Here's how the part is built. I have some questions about the finished solid (model axes, mm). A direction names the side the tool comes from. Give positions to 0.01 mm unless a question says otherwise; leave off trailing zeros. Write each loop counter-clockwise with the first axis right and the second up, starting at its lowest first coordinate (ties: lowest second). Pieces come first, ordered by that corner, then holes. Notation, with made-up numbers: (27, -3) -> (46, -3) arc R25 ccw to (46, 18) -> close; hole circle Ø9 at (33.5, -4). An arc over 180 degrees is marked (long way). Use one line per item in the form item = value.
```python
from build123d import *

# Parameters (mm, degrees)
SKETCH_1_R           = 7.83
EXTRUDE_1_DEPTH      = 5.5
EXTRUDE_1_DEPTH_BACK = 5.5
SKETCH_3_R           = 9.5
EXTRUDE_3_DEPTH      = 1.5
SKETCH_4_R           = 9.5
EXTRUDE_4_DEPTH      = 1.5
SKETCH_5_R           = 3
CUT_EXTRUDE_1_DEPTH  = 15
SKETCH_6_R           = 2
CUT_EXTRUDE_2_DEPTH  = 10.5
SKETCH_7_R           = 2
CUT_EXTRUDE_3_DEPTH  = 10.5


with BuildPart() as part:
    # Sketch 1 → Extrude 1 (new body, two sides)
    with BuildSketch(Plane(origin=(0, 0, 0), x_dir=(1, 0, 0), z_dir=(0, 1, 0))) as extrude_1_sk:
        Circle(SKETCH_1_R)
    extrude(amount=EXTRUDE_1_DEPTH)
    extrude(extrude_1_sk.sketch, amount=-EXTRUDE_1_DEPTH_BACK)

    # Sketch 3 → Extrude 3 (add)
    with BuildSketch(Plane.XZ.offset(5.5)):
        Circle(SKETCH_3_R)
    extrude(amount=EXTRUDE_3_DEPTH)

    # Sketch 4 → Extrude 4 (add)
    with BuildSketch(Plane(origin=(0, 5.5, 0), x_dir=(1, 0, 0), z_dir=(0, 1, 0))):
        Circle(SKETCH_4_R)
    extrude(amount=EXTRUDE_4_DEPTH)

    # Sketch 5 → Cut-Extrude 1 (cut, through all)
    with BuildSketch(Plane.XZ.offset(7)):
        Circle(SKETCH_5_R)
    extrude(amount=-CUT_EXTRUDE_1_DEPTH, mode=Mode.SUBTRACT)

    # Sketch 6 → Cut-Extrude 2 (cut, through all)
    with BuildSketch(Plane.XY):
        Circle(SKETCH_6_R)
    extrude(amount=CUT_EXTRUDE_2_DEPTH, mode=Mode.SUBTRACT)

    # Sketch 7 → Cut-Extrude 3 (cut, through all)
    with BuildSketch(Plane(origin=(0, 0, 0), x_dir=(0, 0, -1), z_dir=(1, 0, 0))):
        Circle(SKETCH_7_R)
    extrude(amount=-CUT_EXTRUDE_3_DEPTH, mode=Mode.SUBTRACT)


solid = part.part
```
Q1. If I drill on line 1 along Y through (x, z) = (-4.75, 6.5); line 2 along Y through (x, z) = (0, 7.5); line 3 along Z through (x, y) = (0, -0.5), over which ranges is the centre line in solid material (lowest first)? Write a range as from..to.
Result set:
line_1 = -7..-5.5, 5.5..7
line_2 = -7..-2, 2..7
line_3 = -7.83..-3
Q2. I want a section at D-D, the plane y = -3.75. Write out the boundary of the cut face in (x, z), and give its area (3 significant figures).
Result set:
outline = circle Ø15.66 at (0, 0); hole circle Ø6 at (0, 0)
area = 164 mm2
Q3. I want a section at C-C, the plane x = 2.75. Write out the boundary of the cut face in (y, z), and give its area (3 significant figures).
Result set:
outline = (-7, -9.09) -> (-5.5, -9.09) -> (-5.5, -7.33) -> (5.5, -7.33) -> (5.5, -9.09) -> (7, -9.09) -> (7, -1.2) -> (-7, -1.2) -> close; (-7, 1.2) -> (7, 1.2) -> (7, 9.09) -> (5.5, 9.09) -> (5.5, 7.33) -> (-5.5, 7.33) -> (-5.5, 9.09) -> (-7, 9.09) -> close
area = 182 mm2
Q4. I want a section at A-A, the plane x = 0. Write out the boundary of the cut face in (y, z), and give its area (3 significant figures).
Result set:
outline = (-7, -9.5) -> (-5.5, -9.5) -> (-5.5, -7.83) -> (5.5, -7.83) -> (5.5, -9.5) -> (7, -9.5) -> (7, -3) -> (-7, -3) -> close; (-7, 3) -> (-2, 3) -> (-2, 7.83) -> (-5.5, 7.83) -> (-5.5, 9.5) -> (-7, 9.5) -> close; (2, 3) -> (7, 3) -> (7, 9.5) -> (5.5, 9.5) -> (5.5, 7.83) -> (2, 7.83) -> close
area = 126 mm2
Q5. Which directions (+Z, -Z, +X, -X, +Y, -Y) give clear straight access to the entire face, cutting with the end or side of a thin tool? Please do faces 5 (the face through (-4.994, -0.766, -1.847)), 6 (the face through (-2.24, 7, -2.24)), 7 (the face through (1, -5.5, 8)).
Result set:
face_5 = -X
face_6 = +Z, -Z, +X, -X, +Y
face_7 = none
Q6. If we mould it in two halves opening along X, with no side actions, what happens to faces 1 (the face through (1.384, -0.098, -2.662)), 2 (the face through (1.847, -0.766, 4.997)), 3 (the face through (7.47, 0.08, -2.35)), 4 (the face through (-2.24, -7, 2.24))? For each: +X half, -X half, draft (parallel to the pull), parting line (faces both ways), or undercut.
Result set:
face_1 = undercut
face_2 = undercut
face_3 = parting line
face_4 = draft
Q7. I want a section at B-B, the plane z = 0. Write out the boundary of the cut face in (x, y).
Result set:
outline = (-9.5, -7) -> (-3, -7) -> (-3, -2) -> (-7.83, -2) -> (-7.83, -5.5) -> (-9.5, -5.5) -> close; (-9.5, 5.5) -> (-7.83, 5.5) -> (-7.83, 2) -> (-3, 2) -> (-3, 7) -> (-9.5, 7) -> close; (3, -7) -> (9.5, -7) -> (9.5, -5.5) -> (7.83, -5.5) -> (7.83, 5.5) -> (9.5, 5.5) -> (9.5, 7) -> (3, 7) -> close
Q8. Will these pins go through, and if not, where does the flat tip stop? pin 1 Ø3.5 at (y, z) = (0, 0) entering from -X; pin 2 Ø3 at (x, y) = (-5.5, -2.5) entering from +Z; pin 3 Ø1.5 at (x, y) = (-6, -1) entering from -Z.
Result set:
pin_1 = 2.44
pin_2 = 6.73
pin_3 = -5.81
